Here's how the part is built. I have some questions about the finished solid (model axes, mm). A direction names the side the tool comes from. Coordinates: 2 decimals unless noted, no trailing zeros. Order: outer loops, then holes, each group sorted by start corner. A loop starts at its lowest first (then second) coordinate and runs counter-clockwise, first axis right, second up. Notation, with made-up numbers: (50, 69.5) - (75, 69.5) arc R19 ccw to (75, 103.5) - close; hole circle Ø1 at (62.25, 82). An arc over 180 degrees is marked (long way). Use one line per item in the form item = value. Start each with the question number.
from build123d import *

# Parameters (mm, degrees)
F3_D = 10.3


with BuildPart() as f1:
    # F0 (on Top) → F1 (revolve)
    with BuildSketch(Plane.XY):
        Polygon((0, 25), (0, 0), (44.95, 0), (44.95, 1.8701055199), (44.1626615226, 1.8701055199), (44.1626615226, 3), (43.5877479613, 3), (43.5877479613, 4.5), (44.1626615226, 4.5), (44.1626615226, 22), (42.6626615226, 22), (42.6626615226, 23.5), (44.1626615226, 23.5), (44.1626615226, 25), align=None)
    revolve(axis=Axis((0, 12.5, 0), (0, 1, 0)))

    # F3 (through all)
    with Locations(Plane.XZ):
        with Locations((0, 0)):
            Hole(F3_D / 2)


solid = f1.part
1) Suppose I cut it at D-D, the plane z = 28. List the corners of the cut face in (x, y) for me.
2) I need wall thicknesses on probe 1 along Y at (x, z) = (-20, 38); probe 2 along Z at (x, y) = (0, 14.5); probe 3 along X at (y, z) = (2.25, 2). Which ranges of each line are inside material? Lowest first, please. Write a range as [from, to].
3) Suppose I cut it at B-B, the plane x = 0. List the corners of the cut face in (y, z) for me.
4) If we mould it in two halves opening along Y, with no side actions, what happens to faces 4 (the flat face through (-9, 0, -1)), 5 (the flat face through (33, 3, 29)), 6 (the cylindrical face through (-4.91, 12.68, 1.55)), 7 (the flat face through (-33, 4.5, 29))? For each: pulls with the +Y half, pulls with the -Y half, needs draft (parallel to the pull), parting line crosses it, or undercut.
5) Which directions (+Z, -Z, +X, -X, +Y, -Y) give clear straight access to the entire face, cutting with the end or side of a thin tool? Please do faces 1 (the cylindrical face through (-33.13, 0.95, -30.38)), 2 (the cylindrical face through (-5.55, 22.76, -42.3)), 3 (the flat face through (30, 1.87, 33)).
6) For pin 1 (8 mm diameter, centred on x = 19, z = 32.5, fed in from -Y); pin 2 (3 mm diameter, centred on y = 8.5, z = -30.5, fed in from +X); pin 3 (3 mm diameter, centred on x = 16, y = 5, fed in from -Z); pin 4 (5 mm diameter, centred on y = 22, z = -2, fed in from -X), each with a flat end and sliding along its axis, tell me the tip position at first contact or that it passes through.
7) Suppose I cut it at C-C, the plane y = 11.5. List the corners of the cut face in (x, z) for me.
8) Suppose I cut it at A-A, the plane z = 0. List the corners of the cut face in (x, y) for me, then the cut area to 3 significant figures.
From the geometry:
q1.outline = (-35.16, 0) - (35.16, 0) - (35.16, 1.87) - (34.15, 1.87) - (34.15, 3) - (33.4, 3) - (33.4, 4.5) - (34.15, 4.5) - (34.15, 22) - (32.19, 22) - (32.19, 23.5) - (34.15, 23.5) - (34.15, 25) - (-34.15, 25) - (-34.15, 23.5) - (-32.19, 23.5) - (-32.19, 22) - (-34.15, 22) - (-34.15, 4.5) - (-33.4, 4.5) - (-33.4, 3) - (-34.15, 3) - (-34.15, 1.87) - (-35.16, 1.87) - close
q2.probe_1 = [0, 22], [23.5, 25]
q2.probe_2 = [-44.16, -5.15], [5.15, 44.16]
q2.probe_3 = [-44.12, -4.75], [4.75, 44.12]
q3.outline = (0, -44.95) - (1.87, -44.95) - (1.87, -44.16) - (3, -44.16) - (3, -43.59) - (4.5, -43.59) - (4.5, -44.16) - (22, -44.16) - (22, -42.66) - (23.5, -42.66) - (23.5, -44.16) - (25, -44.16) - (25, -5.15) - (0, -5.15) - close; (0, 5.15) - (25, 5.15) - (25, 44.16) - (23.5, 44.16) - (23.5, 42.66) - (22, 42.66) - (22, 44.16) - (4.5, 44.16) - (4.5, 43.59) - (3, 43.59) - (3, 44.16) - (1.87, 44.16) - (1.87, 44.95) - (0, 44.95) - close
q4.face_4 = pulls with the -Y half
q4.face_5 = undercut
q4.face_6 = needs draft
q4.face_7 = undercut
q5.face_1 = +Y, -Y
q5.face_2 = none
q5.face_3 = +Y
q6.pin_1 = 0
q6.pin_2 = 33.31
q6.pin_3 = -41.71
q6.pin_4 = -44.16
q7.outline = circle Ø88.33 at (0, 0); hole circle Ø10.3 at (0, 0)
q8.outline = (-44.95, 0) - (-5.15, 0) - (-5.15, 25) - (-44.16, 25) - (-44.16, 23.5) - (-42.66, 23.5) - (-42.66, 22) - (-44.16, 22) - (-44.16, 4.5) - (-43.59, 4.5) - (-43.59, 3) - (-44.16, 3) - (-44.16, 1.87) - (-44.95, 1.87) - close; (5.15, 0) - (44.95, 0) - (44.95, 1.87) - (44.16, 1.87) - (44.16, 3) - (43.59, 3) - (43.59, 4.5) - (44.16, 4.5) - (44.16, 22) - (42.66, 22) - (42.66, 23.5) - (44.16, 23.5) - (44.16, 25) - (5.15, 25) - close
q8.area = 1,950 mm2
